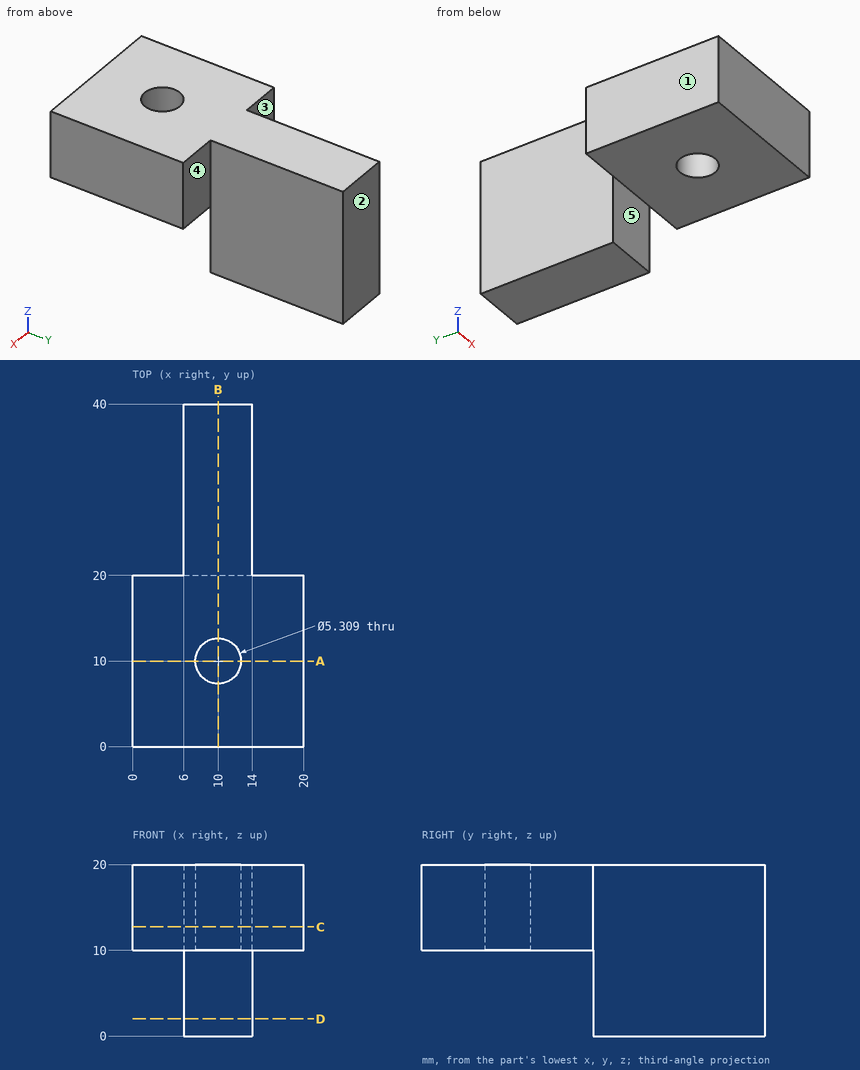
Answer from the drawing. Dimensions are ordinates in mm from the lowest x, y and z of the part. A direction names the side the tool comes from. Give positions to 0.01 mm unless a question says otherwise; leave off trailing zeros. Order: outer loops, then holes, each group sorted by start corner. A loop starts at its lowest first (then second) coordinate and runs counter-clockwise, first axis right, second up.
(1) Find section D-D (z = 2). Give the vertices of the cut face in (x, y), plus the area to 3 significant figures.
(2) Find section B-B (x = 10). Give the vertices of the cut face in (y, z) (1 decimal), plus the area to 3 significant figures.
(3) Straight lines are drawn through the part: L1, parallel to Y at x = 10, z = 15.75 (1 decimal); L2, parallel to X at y = 20.5, z = 16.75; L3, parallel to Y at x = 8.75, z = 3.5. For each, find the intervals that lie inside material, in ascending order.
(4) Given pin 1 (10 mm diameter, centred on y = 32, z = 6.5, fed in from -X); pin 2 (5 mm diameter, centred on x = 2, z = 16, fed in from +Y); pin 3 (12 mm diameter, centred on y = 6.5, z = 3.5, fed in from -X); pin 4 (2.5 mm diameter, centred on x = 9.5, z = 3.5, fed in from -Y), each flat-ended and moving along its own axis, determine where each tip first touches the part or whether it passes through.
(5) Find section A-A (y = 10). Give the vertices of the cut face in (x, z) (1 decimal), plus the area to 3 significant figures.
(6) Find section C-C (z = 12.75). Give the vertices of the cut face in (x, y) (1 decimal), plus the area to 3 significant figures.
(7) For the marked faces 1, 2, 3, 4 and 5, determine the directions among +Z, -Z, +X, -X, +Y, -Y from which every point of the face is accessible in a straight line to the end or side of a thin tool.
Result sheet:
1. outline: (6, 20) - (14, 20) - (14, 40) - (6, 40) - close
1. area: 160 mm2
2. outline: (0, 10) - (7.3, 10) - (7.3, 20) - (0, 20) - close; (12.7, 10) - (20, 10) - (20, 0) - (40, 0) - (40, 20) - (12.7, 20) - close
2. area: 547 mm2
3. L1: y = 0 to 7.3, 12.7 to 40
3. L2: x = 6 to 14
3. L3: y = 20 to 40
4. pin 1: stops at x = 6
4. pin 2: stops at y = 20
4. pin 3: passes through
4. pin 4: stops at y = 20
5. outline: (0, 10) - (7.3, 10) - (7.3, 20) - (0, 20) - close; (12.7, 10) - (20, 10) - (20, 20) - (12.7, 20) - close
5. area: 147 mm2
6. outline: (0, 0) - (20, 0) - (20, 20) - (14, 20) - (14, 40) - (6, 40) - (6, 20) - (0, 20) - close; hole circle Ø5.3 at (10, 10)
6. area: 538 mm2
7. face 1: +Z, -Z, -X, +Y, -Y
7. face 2: +Z, -Z, +X, -X, +Y
7. face 3: +Z, -Z, -X, +Y
7. face 4: +Z, -Z, +X, +Y
7. face 5: -Z, +X, -X, -Y
